Work out the finished part from the listing and answer in its coordinate system (mm). Coordinates: 2 decimals unless noted, no trailing zeros. Write each loop counter-clockwise with the first axis right and the second up, starting at its lowest first coordinate (ties: lowest second). Pieces come first, ordered by that corner, then holes. Notation, with made-up numbers: M 63,21 L 97,21 A15 ccw 97,25 Z; hole C 50,42.5 d11. An arc over 180 degrees is marked long. Use CSV: the item, a comma, the result in double quotes.
from build123d import *

# Parameters (mm, degrees)
SKETCH_1_R      = 50
SKETCH_1_R_2    = 1.5
SKETCH_1_R_3    = 1.25
SKETCH_1_R_4    = 5
SKETCH_1_R_5    = 2.5
EXTRUDE_1_DEPTH = 5


with BuildPart() as part:
    # 草图1 → 凸台-拉伸1 (new body)
    with BuildSketch(Plane.XY):
        Circle(SKETCH_1_R)
        with Locations((0, 44.5)):
            Circle(SKETCH_1_R_2, mode=Mode.SUBTRACT)
        with Locations((44.5, 0)):
            Circle(SKETCH_1_R_2, mode=Mode.SUBTRACT)
        with Locations((0, -44.5)):
            Circle(SKETCH_1_R_2, mode=Mode.SUBTRACT)
        with Locations((-44.5, 0)):
            Circle(SKETCH_1_R_2, mode=Mode.SUBTRACT)
        with Locations((0, 7.5)):
            Circle(SKETCH_1_R_3, mode=Mode.SUBTRACT)
        with Locations((5.303300859, 5.303300859)):
            Circle(SKETCH_1_R_3, mode=Mode.SUBTRACT)
        with Locations((7.5, 0)):
            Circle(SKETCH_1_R_3, mode=Mode.SUBTRACT)
        with Locations((5.303300859, -5.303300859)):
            Circle(SKETCH_1_R_3, mode=Mode.SUBTRACT)
        with Locations((0, -7.5)):
            Circle(SKETCH_1_R_3, mode=Mode.SUBTRACT)
        with Locations((-5.303300859, -5.303300859)):
            Circle(SKETCH_1_R_3, mode=Mode.SUBTRACT)
        with Locations((-7.5, 0)):
            Circle(SKETCH_1_R_3, mode=Mode.SUBTRACT)
        with Locations((-5.303300859, 5.303300859)):
            Circle(SKETCH_1_R_3, mode=Mode.SUBTRACT)
        Circle(SKETCH_1_R_4, mode=Mode.SUBTRACT)
        with Locations((-10.253048327, 32.173358544)):
            Circle(SKETCH_1_R_5, mode=Mode.SUBTRACT)
        with Locations((-32.173358544, 10.253048327)):
            Circle(SKETCH_1_R_5, mode=Mode.SUBTRACT)
        with Locations(Location((10.253048327, 32.173358544, 0), (0, 0, 180))):
            Circle(SKETCH_1_R_5, mode=Mode.SUBTRACT)
        with Locations(Location((32.173358544, 10.253048327, 0), (0, 0, 180))):
            Circle(SKETCH_1_R_5, mode=Mode.SUBTRACT)
        with Locations((-17.5, -30)):
            Circle(SKETCH_1_R_5, mode=Mode.SUBTRACT)
        with Locations((17.5, -30)):
            Circle(SKETCH_1_R_5, mode=Mode.SUBTRACT)
    extrude(amount=EXTRUDE_1_DEPTH)


solid = part.part
Item 1: The part is cut by section B-B (x = -44.5). Write down the section's boundary in (y, z), then the cut area to 3 significant figures.
Answer:
outline,"M -22.8,0 L -1.5,0 L -1.5,5 L -22.8,5 Z; M 1.5,0 L 22.8,0 L 22.8,5 L 1.5,5 Z"
area,"213 mm2"
Item 2: The part is cut by section C-C (z = 2.45). Count the separate pieces of the cut face and the enclosed holes in it, then the cut area to 3 significant figures.
Answer:
separate pieces,"1"
enclosed holes,"19"
area,"7,590 mm2"
Item 3: Consider probe 1 along Y at (x, z) = (0, 0.6); probe 2 along X at (y, z) = (1, 4.25); probe 3 along X at (y, z) = (-29, 1.8). Determine where each line is inside the solid, lowest interval first.
Answer:
probe 1,"y = -50 to -46, -43 to -8.75, -6.25 to -5, 5 to 6.25, 8.75 to 43, 46 to 50"
probe 2,"x = -49.99 to -45.62, -43.38 to -8.25, -6.75 to -4.9, 4.9 to 6.75, 8.25 to 43.38, 45.62 to 49.99"
probe 3,"x = -40.73 to -19.79, -15.21 to 15.21, 19.79 to 40.73"
Item 4: The part is cut by section A-A (y = 0). Write down the section's boundary in (x, z).
Answer:
outline,"M -50,0 L -46,0 L -46,5 L -50,5 Z; M -43,0 L -8.75,0 L -8.75,5 L -43,5 Z; M -6.25,0 L -5,0 L -5,5 L -6.25,5 Z; M 5,0 L 6.25,0 L 6.25,5 L 5,5 Z; M 8.75,0 L 43,0 L 43,5 L 8.75,5 Z; M 46,0 L 50,0 L 50,5 L 46,5 Z"
Item 5: Given pin 1 (3.5 mm diameter, centred on x = 0, y = -44.5, fed in from -Z); pin 2 (1.5 mm diameter, centred on x = 36.5, z = 1.5, fed in from -Y); pin 3 (1 mm diameter, centred on x = 28.5, z = 2, fed in from +Y), each flat-ended and moving along its own axis, determine where each tip first touches the part or whether it passes through.
Answer:
pin 1,"stops at z = 0"
pin 2,"stops at y = -34.96"
pin 3,"stops at y = 41.42"
Item 6: For a pull along Y with two mould halves and no side action, classify faces 1 (the face through (-10.79, 29.73, 2.46)), 2 (the face through (47.69, 15.02, 2.46)), 3 (the face through (-1, -10, 5)) as released by +Y, released by -Y, zero draft, split by the parting line, or undercut.
Answer:
face 1,"undercut"
face 2,"split by the parting line"
face 3,"zero draft"
